from build123d import *

# Parameters (mm, degrees)
F0_R     = 74.008628
F1_DEPTH = 309.88
F2_R     = 69.983842
F3_DEPTH = 415.798
F4_R     = 20.290175
F5_DEPTH = 138.938
F6_DEPTH = 7.62
F7_W     = 139.15725
F7_H     = 11.103896
F8_DEPTH = 97.282


with BuildPart() as f1:
    # F0 (on Top) → F1 (new body)
    with BuildSketch(Plane.XY):
        Circle(F0_R)
    extrude(amount=F1_DEPTH)

    # F2 (on face) → F3 (cut)
    with BuildSketch(Plane.XY.offset(309.88)):
        Circle(F2_R)
    extrude(amount=-F3_DEPTH, mode=Mode.SUBTRACT)

    # F4 (on Right) → F5 (cut)
    with BuildSketch(Plane.YZ):
        with Locations((0, 207.585201)):
            Circle(F4_R)
    extrude(amount=-F5_DEPTH, mode=Mode.SUBTRACT)

    # F0 (on Top) → F6 (join)
    with BuildSketch(Plane.XY):
        Circle(F0_R)
    extrude(amount=-F6_DEPTH)

    # F7 (on Right) → F8 (cut)
    with BuildSketch(Plane.YZ):
        Rectangle(F7_W, F7_H)
    extrude(amount=F8_DEPTH, mode=Mode.SUBTRACT)


solid = f1.part
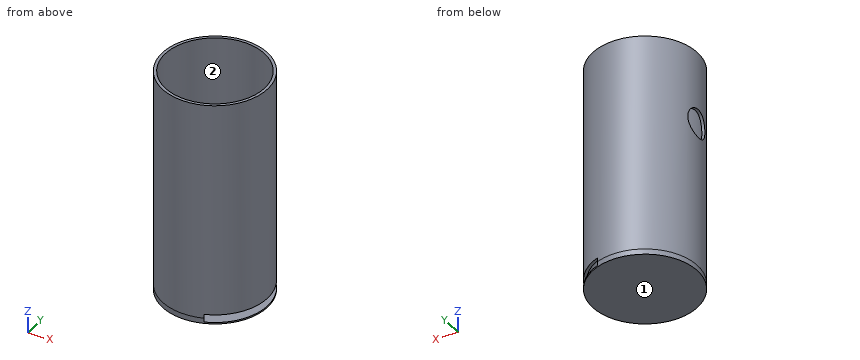
Here's how the part is built. I have some questions about the finished solid (model axes, mm). Face numbers are marked on the shaded views. Round coordinates to 2 decimals unless told otherwise and drop trailing zeros. Order: outer loops, then holes, each group sorted by start corner. A loop starts at its lowest first (then second) coordinate and runs counter-clockwise, first axis right, second up. Notation, with made-up numbers: (-37, 54) -> (3, 54) arc R20 ccw to (3, 79) -> close; hole circle Ø11 at (31.25, 6.25). An arc over 180 degrees is marked (long way). Return JSON: item names as keys, results as strings.
Q1. For pin 1 Ø10 at (x, y) = (-6, -14.5) entering from +Z; pin 2 Ø1.5 at (y, z) = (8, 248.5) entering from +X; pin 3 Ø1.7 at (y, z) = (-14.5, -2.5) entering from +X, each with a flat end and sliding along its axis, tell me the tip position at first contact or that it passes through.
Filled sheet:
{"pin 1": "stops at z = 0", "pin 2": "stops at x = 73.65", "pin 3": "stops at x = 0"}
Q2. If we section it at B-B on x = 45.5: List the corners of the cut face in (y, z) for me.
Filled sheet:
{"outline": "(-58.37, -7.62) -> (58.37, -7.62) -> (58.37, -5.55) -> (-58.37, -5.55) -> close; (-58.37, 5.55) -> (-53.17, 5.55) -> (-53.17, 309.88) -> (-58.37, 309.88) -> close; (53.17, 5.55) -> (58.37, 5.55) -> (58.37, 309.88) -> (53.17, 309.88) -> close"}
Q3. If we section it at D-D on z = 28: List the corners of the cut face in (x, y) for me.
Filled sheet:
{"outline": "circle Ø148.02 at (0, 0); hole circle Ø139.97 at (0, 0)"}
Q4. If we section it at A-A on y = 0: List the corners of the cut face in (x, z) for me.
Filled sheet:
{"outline": "(-74.01, -7.62) -> (74.01, -7.62) -> (74.01, -5.55) -> (0, -5.55) -> (0, 0) -> (-69.98, 0) -> (-69.98, 187.3) -> (-74.01, 187.3) -> close; (-74.01, 227.88) -> (-69.98, 227.88) -> (-69.98, 309.88) -> (-74.01, 309.88) -> close; (69.98, 5.55) -> (74.01, 5.55) -> (74.01, 309.88) -> (69.98, 309.88) -> close"}
Q5. I need wall thicknesses on line 1 along Z through (x, y) = (65.5, -32); line 2 along Y through (x, z) = (0, 200); line 3 along Y through (x, z) = (-2, 190). Which ranges of each line are inside material? Lowest first, please. Write a range as from..to.
Filled sheet:
{"line 1": "z = -7.62..-5.55, 5.55..309.88", "line 2": "y = -74.01..-69.98, 69.98..74.01", "line 3": "y = -73.98..-69.96, 69.96..73.98"}
Q6. If we mould it in two halves opening along Y, with no side actions, what happens to the marked faces 1 and 2? For each: released by +Y, released by -Y, zero draft, split by the parting line, or undercut.
Filled sheet:
{"face 1": "zero draft", "face 2": "undercut"}
Q7. If we section it at C-C on y = 36: List the corners of the cut face in (x, z) for me, plus the area to 3 significant figures.
Filled sheet:
{"outline": "(-64.66, -7.62) -> (64.66, -7.62) -> (64.66, -5.55) -> (0, -5.55) -> (0, 0) -> (-60.01, 0) -> (-60.01, 309.88) -> (-64.66, 309.88) -> close; (60.01, 5.55) -> (64.66, 5.55) -> (64.66, 309.88) -> (60.01, 309.88) -> close", "area": "3,480 mm^2"}
